Work out the finished part from the listing and answer in its coordinate system (mm). Face numbers are marked on the shaded views. A direction names the side the tool comes from. Round coordinates to 2 decimals unless told otherwise and drop trailing zeros. Order: outer loops, then holes, each group sorted by start corner. A loop starts at its lowest first (then second) coordinate and runs counter-clockwise, first axis right, second up. Notation, with made-up numbers: M 56.5,22.5 L 61.5,22.5 A18 ccw 61.5,55.5 Z; hole C -16,-24 d10. An arc over 180 degrees is marked long. Answer as a JSON object with one key per item and string values. Group by question number.
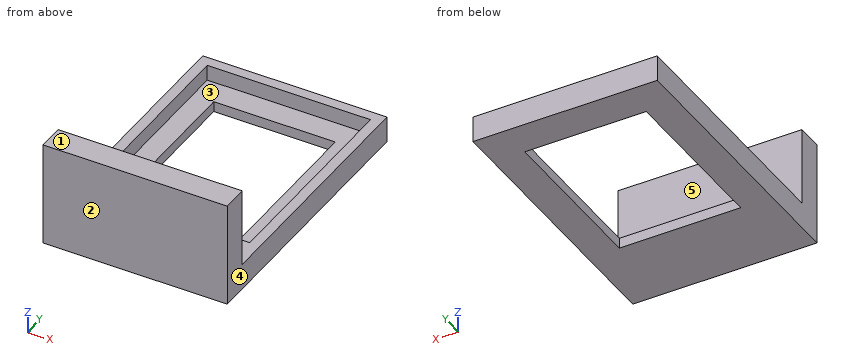
from build123d import *

# Parameters (mm, degrees)
F0_W     = 22.352
F0_H     = 30.734
F0_W_2   = 14.732
F0_H_2   = 20.066
F1_DEPTH = 3.175
F2_W     = 19.812
F2_H     = 25.654
F2_W_2   = 14.732
F2_H_2   = 20.066
F3_DEPTH = 1.905
F0_H_3   = 3.175
F4_DEPTH = 12.7


with BuildPart() as f1:
    # F0 (on Top) → F1 (new body)
    with BuildSketch(Plane.XY):
        with Locations((11.176, 15.367)):
            Rectangle(F0_W, F0_H)
        with Locations((11.176, 16.383)):
            Rectangle(F0_W_2, F0_H_2, mode=Mode.SUBTRACT)
    extrude(amount=F1_DEPTH)

    # F2 (on face) → F3 (cut)
    with BuildSketch(Plane.XY.offset(3.175)):
        with Locations((11.176, 16.637)):
            Rectangle(F2_W, F2_H)
        with Locations((11.176, 16.383)):
            Rectangle(F2_W_2, F2_H_2, mode=Mode.SUBTRACT)
    extrude(amount=-F3_DEPTH, mode=Mode.SUBTRACT)

    # F0 (on Top) → F4 (join)
    with BuildSketch(Plane.XY):
        with Locations((11.176, -1.5875)):
            Rectangle(F0_W, F0_H_3)
    extrude(amount=F4_DEPTH)


solid = f1.part
Item 1: Find section D-D (y = 1.5). Give the vertices of the cut face in (x, z) (3 decimals), and give its area (3 significant figures).
Item 2: Find section C-C (z = 10.25). Give the vertices of the cut face in (x, y) (3 decimals), and give its area (3 significant figures).
Item 3: Each of these flat-tipped pins is pushed along its axis until it touches: pin 1 (10 mm diameter, centred on x = 13, y = 24, fed in from +Z); pin 2 (5 mm diameter, centred on x = 16.5, z = 8, fed in from +Y); pin 3 (4 mm diameter, centred on x = 17, y = 3, fed in from +Z) (3 decimals). Where does it stop, or does it pass through?
Item 4: Find section B-B (y = 17). Give the vertices of the cut face in (x, z) (3 decimals), and give its area (3 significant figures).
Item 5: Consider L1, parallel to Y at x = 3.25, z = 1.5 (3 decimals); L2, parallel to X at y = 12.5, z = 2.25; L3, parallel to Y at x = 19, z = 7.5 (3 decimals). Determine where each line is inside the solid, lowest interval first.
Item 6: A tool of negligible diameter and unlimited length cuts with its end or side. For the marked faces 4 and 5, from which of +Z, -Z, +X, -X, +Y, -Y can it reach the whole face along a straight path? Write none if from no direction.
Item 7: The mould has two halves that part along Y. Classify the marked faces 1, 2 and 3: +Y half, -Y half, draft (parallel to the pull), parting line (faces both ways), or undercut.
Item 8: Find section A-A (x = 12.25). Give the vertices of the cut face in (y, z) (3 decimals).
Responses:
{
 "1": {"outline": "M 0,0 L 22.352,0 L 22.352,3.175 L 0,3.175 Z", "area": "71.0 mm^2"},
 "2": {"outline": "M 0,-3.175 L 22.352,-3.175 L 22.352,0 L 0,0 Z", "area": "71.0 mm^2"},
 "3": {"pin 1": "stops at z = 1.27", "pin 2": "stops at y = 0", "pin 3": "stops at z = 3.175"},
 "4": {"outline": "M 0,0 L 3.81,0 L 3.81,1.27 L 1.27,1.27 L 1.27,3.175 L 0,3.175 Z; M 18.542,0 L 22.352,0 L 22.352,3.175 L 21.082,3.175 L 21.082,1.27 L 18.542,1.27 Z", "area": "14.5 mm^2"},
 "5": {"L1": "y = -3.175 to 3.81, 29.464 to 30.734", "L2": "x = 0 to 1.27, 21.08 to 22.35", "L3": "y = -3.175 to 0"},
 "6": {"face 4": "+Z, -Z, +X, +Y, -Y", "face 5": "+Z, +X, -X, +Y"},
 "7": {"face 1": "draft", "face 2": "-Y half", "face 3": "undercut"},
 "8": {"outline": "M -3.175,0 L 6.35,0 L 6.35,1.27 L 3.81,1.27 L 3.81,3.175 L 0,3.175 L 0,12.7 L -3.175,12.7 Z; M 26.416,0 L 30.734,0 L 30.734,3.175 L 29.464,3.175 L 29.464,1.27 L 26.416,1.27 Z"}
}
